Here's how the part is built. I have some questions about the finished solid (model axes, mm). A direction names the side the tool comes from. Round coordinates to 2 decimals unless told otherwise and drop trailing zeros. Loops run counter-clockwise (first coordinate to the right, second up) from the corner with the lowest first, then second, coordinate; pieces in that order, holes last. Notation, with made-up numbers: M 46,8.5 L 100,8.5 A9 cw 100,15.5 Z; hole C 62,-35.75 d9. An arc over 180 degrees is marked long. Answer as a JSON object with one key per item and string values.
from build123d import *

# Parameters (mm, degrees)
F0_W     = 150
F0_H     = 150
F1_DEPTH = 70
F2_T     = -25
F3_R     = 44.99999


# Not quite as in the source:
# - a fillet or chamfer is up to 0.001 mm smaller than in the source, because OpenCascade refuses the exact size


with BuildPart() as f1:
    # F0 (on Top) → F1 (new body)
    with BuildSketch(Plane.XY):
        Rectangle(F0_W, F0_H)
    extrude(amount=F1_DEPTH)

    # F2
    f2_openings = [f1.faces().sort_by_distance(p)[0] for p in [
        (0, 0, 70),
    ]]
    offset(amount=F2_T, openings=f2_openings)

    # F3 (radius 45 in the source; OpenCascade refuses exactly that, so slightly less here)
    f3_edges = [f1.edges().sort_by_distance(p)[0] for p in [
        (0, 50, 25),
        (-50, 0, 25),
        (50, 0, 25),
        (0, -50, 25),
        (50, -50, 47.5),
        (50, 50, 47.5),
        (-50, 50, 47.5),
        (-50, -50, 47.5),
    ]]
    fillet(f3_edges, radius=F3_R)


solid = f1.part
Item 1: We'd pull the mould along X, two halves only. Please class faces 1 (the face through (0.07, 37.168, 38.532)), 2 (the face through (-75, -1, 35)), 3 (the face through (-1, -75, 35)), 4 (the face through (0, 0, 25)): +X half, -X half, draft (parallel to the pull), parting line (faces both ways), or undercut.
Solution:
{"face 1": "undercut", "face 2": "-X half", "face 3": "draft", "face 4": "undercut"}
Item 2: For faces 5 (the face through (-1, 75, 35)), 6 (the face through (37.168, 0.07, 38.532)), which set-ups out of +Z, -Z, +X, -X, +Y, -Y let a thin tool reach every point of the face, with its end or its side?
Solution:
{"face 5": "+Z, -Z, +X, -X, +Y", "face 6": "+Z"}
Item 3: I want a section at D-D on z = 52.5. List the corners of the cut face in (x, y) for me, plus the area to 3 significant figures.
Solution:
{"outline": "M -75,-75 L 75,-75 L 75,75 L -75,75 Z; hole M -46.46,-5 A41.46 ccw -5,-46.46 L 5,-46.46 A41.46 ccw 46.46,-5 L 46.46,5 A41.46 ccw 5,46.46 L -5,46.46 A41.46 ccw -46.46,5 Z", "area": "15,300 mm2"}
Item 4: I want a section at A-A on z = 65.5. List the corners of the cut face in (x, y) for me, plus the area to 3 significant figures.
Solution:
{"outline": "M -75,-75 L 75,-75 L 75,75 L -75,75 Z; hole M -49.77,-5 A44.77 ccw -5,-49.77 L 5,-49.77 A44.77 ccw 49.77,-5 L 49.77,5 A44.77 ccw 5,49.77 L -5,49.77 A44.77 ccw -49.77,5 Z", "area": "14,300 mm2"}
Item 5: For P1, Ø8, axis at x = 1.5, y = 2.5, coming from the +Z side (3 decimals), with a flat end and sliding along its axis, tell me the tip position at first contact or that it passes through.
Solution:
{"P1": "stops at z = 25.025"}
Item 6: If I drill on L1, parallel to X at y = 36, z = 50; L2, parallel to X at y = -32, z = 58; L3, parallel to Y at x = 4.5, z = 58.5, over which ranges is the centre line in solid material (lowest first)? Write a range as from..to.
Solution:
{"L1": "x = -75..-30.77, 30.77..75", "L2": "x = -75..-38.94, 38.94..75", "L3": "y = -75..-48.51, 48.51..75"}
